Design review of the part built by this model. Coordinates are the model's own, in mm. Face numbers are marked on the shaded views. Coordinates: 2 decimals unless noted, no trailing zeros. Loops run counter-clockwise (first coordinate to the right, second up) from the corner with the lowest first, then second, coordinate; pieces in that order, holes last. Notation, with made-up numbers: (61, -32.75) - (100, -32.75) arc R27 cw to (100, -13.75) - close; hole circle Ø8 at (30, -9.5). An arc over 180 degrees is marked (long way). Answer in a Markdown table with one row per item. Add a question column.
(1) We need section B-B, the plane x = 136. Write out the cut boundary in (y, z), plus the area to 3 significant figures.
(2) To check wall thickness, follow L1, parallel to X at y = 159, z = 9.5; L2, parallel to Y at x = 31, z = 1.25; L3, parallel to X at y = 155, z = 9.25. State the ranges of each line that lie inside material, in increasing order. Write a range as [from, to].
(3) Clearance check with flat-ended pins moving along their axes: pin 1 (3 mm diameter, centred on x = 73, z = 3, fed in from +Y); pin 2 (6 mm diameter, centred on x = 129, z = 5.5, fed in from -Y); pin 3 (1 mm diameter, centred on x = 172, z = 1.5, fed in from -Y). State where each tip first meets the part, or that it passes through.
(4) The part is to be moulded in two halves that separate along Y. For the marked faces 1, 2 and 3, say which applies: released by +Y, released by -Y, zero draft, split by the parting line, or undercut.
(5) We need section A-A, the plane x = 98. Write out the cut boundary in (y, z).
from build123d import *

# Parameters (mm, degrees)
PAD_DEPTH = 10


with BuildPart() as part:
    # Sketch → Pad (new body)
    with BuildSketch(Plane(origin=(0, 0, 0), x_dir=(0.866025, 0.5, 0), z_dir=(0, 0, 1))):
        with BuildLine():
            Line((301.034851, -0.014674), (299.858856, 0.018))
            Line((299.858856, 0.018), (298.818, 0.072))
            Line((298.818, 0.072), (297.342, 0.183))
            Line((297.342, 0.183), (295.287, 0.363))
            Line((295.287, 0.363), (292.659, 0.621))
            Line((292.659, 0.621), (289.467, 0.957))
            Line((289.467, 0.957), (285.723, 1.368))
            Line((285.723, 1.368), (281.445, 1.851))
            Line((281.445, 1.851), (276.648, 2.403))
            Line((276.648, 2.403), (273.162811, 3.038512))
            Line((273.162811, 34.144974), (273.162811, 3.038512))
            Line((273.162811, 34.144974), (166.153931, 34.144974))
            ThreePointArc((166.153931, 34.144974), (148.85588, 28.812612), (132.373183, 21.330808))
            Line((132.373183, 21.330808), (121.893, 22.038))
            Line((121.893, 22.038), (112.698, 22.761))
            Line((112.698, 22.761), (103.647, 23.322))
            Line((103.647, 23.322), (94.782, 23.703))
            Line((94.782, 23.703), (86.133, 23.886))
            Line((86.133, 23.886), (77.736, 23.856))
            Line((77.736, 23.856), (69.627, 23.607))
            Line((69.627, 23.607), (61.833, 23.127))
            Line((61.833, 23.127), (54.387, 22.419))
            Line((54.387, 22.419), (47.319, 21.486))
            Line((47.319, 21.486), (40.656, 20.34))
            Line((40.656, 20.34), (34.422, 18.996))
            Line((34.422, 18.996), (28.647, 17.472))
            Line((28.647, 17.472), (23.352, 15.798))
            Line((23.352, 15.798), (18.555, 13.998))
            Line((18.555, 13.998), (14.277, 12.105))
            Line((14.277, 12.105), (10.533, 10.155))
            Line((10.533, 10.155), (7.341, 8.184))
            Line((7.341, 8.184), (4.713, 6.246))
            Line((4.713, 6.246), (2.658, 4.41))
            Line((2.658, 4.41), (1.182, 2.745))
            Line((1.182, 2.745), (0.297, 1.281))
            Line((0.297, 1.281), (0, 0))
            Line((0, 0), (0.297, -1.17))
            Line((0.297, -1.17), (1.182, -2.301))
            Line((1.182, -2.301), (2.886778, -4.059651))
            ThreePointArc((2.886778, -4.059651), (12.612237, -20.403463), (27.278178, -32.511927))
            Line((27.278178, -32.511927), (256.779602, -32.435658))
            ThreePointArc((272.568004, -3.393518), (260.687772, -15.747631), (256.779602, -32.435658))
            Line((272.568004, -3.393518), (276.648, -2.355))
            Line((276.648, -2.355), (281.445, -1.827))
            Line((281.445, -1.827), (285.723, -1.359))
            Line((285.723, -1.359), (289.467, -0.954))
            Line((289.467, -0.954), (292.659, -0.618))
            Line((292.659, -0.618), (295.287, -0.363))
            Line((295.287, -0.363), (297.342, -0.183))
            Line((297.342, -0.183), (298.818, -0.072))
            Line((298.818, -0.072), (299.703, -0.018))
            Line((299.703, -0.018), (301.034851, -0.014674))
        make_face()
    extrude(amount=PAD_DEPTH)


solid = part.part
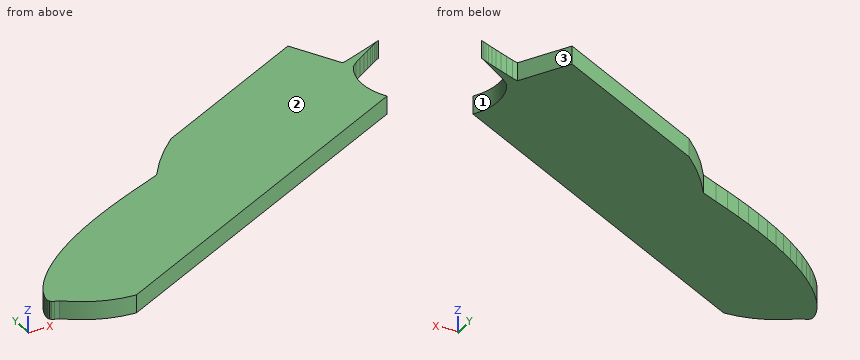
Responses:
| question | item | result |
|---|---|---|
| 1 | outline | (41.02, 0) - (117.95, 0) - (117.95, 10) - (41.02, 10) - close |
| 1 | area | 769 mm2 |
| 2 | L1 | x = [207.11, 223.62] |
| 2 | L2 | y = [-13.85, 42.85] |
| 2 | L3 | x = [200.18, 225.93] |
| 3 | pin 1 | stops at y = 70.14 |
| 3 | pin 2 | stops at y = 35.24 |
| 3 | pin 3 | stops at y = 61.53 |
| 4 | face 1 | undercut |
| 4 | face 2 | zero draft |
| 4 | face 3 | released by +Y |
| 5 | outline | (19.06, 0) - (81.73, 0) - (81.73, 10) - (19.06, 10) - close |
